Job drawing, mm, ordinate dimensions from the low corner. One solid piece. Give positions to 0.01 mm unless a question says otherwise; leave off trailing zeros. Order: outer loops, then holes, each group sorted by start corner. A loop starts at its lowest first (then second) coordinate and runs counter-clockwise, first axis right, second up. Notation, with made-up numbers: M -28.5,16.25 L -11.5,16.25 A15 ccw -11.5,31.25 Z; hole C 54,41.5 d7. An arc over 180 degrees is marked long. One line per question, with ' | ' between items.
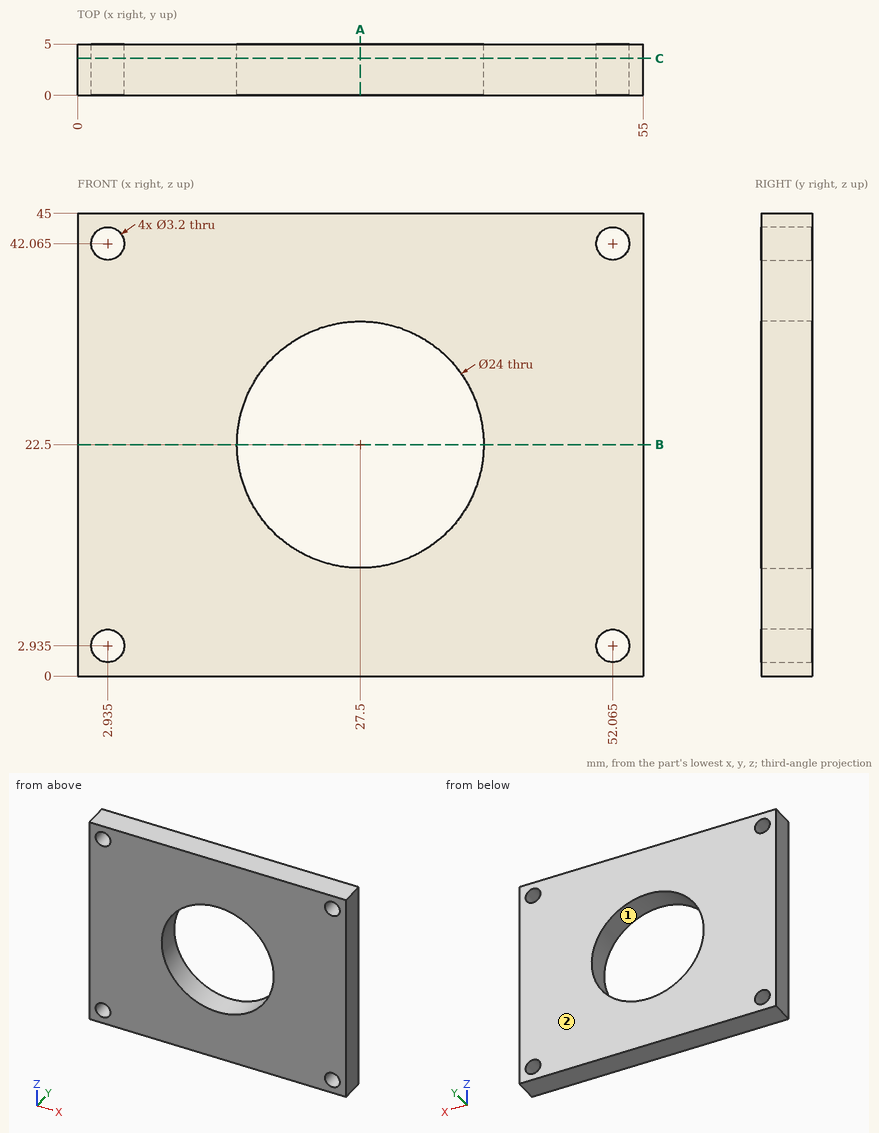
1. Slice it at B-B on z = 22.5. Give the cut face in (x, y).
Worked out:
outline: M 0,0 L 15.5,0 L 15.5,5 L 0,5 Z; M 39.5,0 L 55,0 L 55,5 L 39.5,5 Z
2. Probe L1, parallel to X at y = 1.45, z = 22.5; L2, parallel to X at y = 1.6, z = 3.5; L3, parallel to X at y = 1.4, z = 21. List the from-to ranges inside material, lowest first. Write a range as from..to.
Worked out:
L1: x = 0..15.5, 39.5..55 | L2: x = 0..1.44, 4.43..50.57, 53.56..55 | L3: x = 0..15.59, 39.41..55
3. Mould opens along X. For the marked faces 1 and 2 say: released by +X, released by -X, zero draft, split by the parting line, or undercut.
Worked out:
face 1: undercut | face 2: zero draft
4. Slice it at C-C on y = 3.6. Give the cut face in (x, z) (1 decimal), then the cut area to 3 significant figures.
Worked out:
outline: M 0,0 L 55,0 L 55,45 L 0,45 Z; hole C 2.9,2.9 d3.2; hole C 2.9,42.1 d3.2; hole C 27.5,22.5 d24; hole C 52.1,2.9 d3.2; hole C 52.1,42.1 d3.2 | area: 1,990 mm2
5. Slice it at A-A on x = 27.5. Give the cut face in (y, z), then the cut area to 3 significant figures.
Worked out:
outline: M 0,0 L 5,0 L 5,10.5 L 0,10.5 Z; M 0,34.5 L 5,34.5 L 5,45 L 0,45 Z | area: 105 mm2
